```python
from build123d import *

# Parameters (mm, degrees)
BOSS_EXTRUDE1_DEPTH             = 7.62
SKETCH1_3_R                     = 1.5
BOSS_EXTRUDE2_DEPTH             = 2.54
SKETCH2_W                       = 63.119
SKETCH2_H                       = 7.62
BOSS_EXTRUDE3_DEPTH             = 2.54
BOSS_EXTRUDE3_DIRECTION_2_REACH = 58.274
FILLET1_R                       = 15.24
FILLET2_R                       = 5.08
FILLET3_R                       = 2.54


with BuildPart() as part:
    # Sketch1 → Boss-Extrude1 (new body)
    with BuildSketch(Plane.XY):
        with BuildLine():
            Line((-37.554226409, 19.773329444), (-37.554226409, 16.344329444))
            Line((-37.554226409, 16.344329444), (-8.344226409, 16.344329444))
            ThreePointArc((-8.344226409, 16.344329444), (-0.261995901, 12.996559953), (3.085773591, 4.914329444))
            Line((3.085773591, 4.914329444), (3.085773591, -14.770670556))
            Line((3.085773591, -14.770670556), (-37.554226409, -14.770670556))
            Line((-37.554226409, -14.770670556), (-37.554226409, -21.438170556))
            Line((-37.554226409, -21.438170556), (6.514773591, -21.438170556))
            Line((6.514773591, -21.438170556), (25.564773591, -21.120670556))
            Line((25.564773591, -21.120670556), (6.514773591, -6.642670556))
            Line((6.514773591, -6.642670556), (6.514773591, 4.914329444))
            ThreePointArc((6.514773591, 4.914329444), (2.162673252, 15.421229106), (-8.344226409, 19.773329444))
            Line((-8.344226409, 19.773329444), (-37.554226409, 19.773329444))
        make_face()
    extrude(amount=-BOSS_EXTRUDE1_DEPTH)

    # Sketch1<3> → Boss-Extrude2 (add)
    with BuildSketch(Plane.XY):
        with BuildLine():
            Line((-8.344226409, 16.344329444), (-37.554226409, 16.344329444))
            Line((-37.554226409, 16.344329444), (-37.554226409, -14.770670556))
            Line((-37.554226409, -14.770670556), (3.085773591, -14.770670556))
            Line((3.085773591, -14.770670556), (3.085773591, 4.914329444))
            ThreePointArc((3.085773591, 4.914329444), (-0.261995901, 12.996559953), (-8.344226409, 16.344329444))
        make_face()
        with Locations((-29.732882342, -7.215397763)):
            Circle(SKETCH1_3_R, mode=Mode.SUBTRACT)
        with Locations((-4.332882342, -7.215397763)):
            Circle(SKETCH1_3_R, mode=Mode.SUBTRACT)
        with Locations((-29.710505244, 10.645398587)):
            Circle(SKETCH1_3_R, mode=Mode.SUBTRACT)
        with Locations((-4.310505244, 10.645398587)):
            Circle(SKETCH1_3_R, mode=Mode.SUBTRACT)
    extrude(amount=-BOSS_EXTRUDE2_DEPTH)

    # Sketch2 → Boss-Extrude3 (add)
    with BuildSketch(Plane.XZ.offset(21.438170556)):
        with Locations((-5.994726409, -3.81)):
            Rectangle(SKETCH2_W, SKETCH2_H)
    extrude(amount=BOSS_EXTRUDE3_DEPTH)

    # Boss-Extrude3 direction 2: up to this face of the body (flat: up to its plane)
    boss_extrude3_direction_2_end = Plane(part.part.faces().sort_by_distance((16.039773591, -21.279420556, -3.81))[0])
    # Sketch2 → Boss-Extrude3 direction 2 (add, up to the picked face)
    with BuildSketch(Plane.XZ.offset(21.438170556), mode=Mode.PRIVATE) as boss_extrude3_direction_2_sk1:
        with Locations((-5.994726409, -3.81)):
            Rectangle(SKETCH2_W, SKETCH2_H)
    boss_extrude3_direction_2_tool1 = split(extrude(boss_extrude3_direction_2_sk1.sketch, amount=-BOSS_EXTRUDE3_DIRECTION_2_REACH, mode=Mode.PRIVATE), bisect_by=boss_extrude3_direction_2_end, keep=Keep.BOTH, mode=Mode.PRIVATE)
    add(boss_extrude3_direction_2_tool1.solids().sort_by(Axis((-5.994726, -21.438171, -3.81), (0, 1, 0)))[0])

    # Fillet1
    fillet1_edges = [part.edges().sort_by_distance(p)[0] for p in [
        (-37.554226409, 19.773329444, -3.81),
        (-37.554226409, -23.978170556, -3.81),
    ]]
    fillet(fillet1_edges, radius=FILLET1_R)

    # Fillet2
    fillet2_edges = [part.edges().sort_by_distance(p)[0] for p in [
        (25.564773591, -21.120670556, -3.81),
    ]]
    fillet(fillet2_edges, radius=FILLET2_R)

    # Fillet3
    fillet3_edges = [part.edges().sort_by_distance(p)[0] for p in [
        (6.514773591, -6.642670556, -3.81),
    ]]
    fillet(fillet3_edges, radius=FILLET3_R)


solid = part.part
```
The model under review builds one solid part; all positions refer to its coordinate system, in mm. A direction names the side the tool comes from. Give positions to 0.01 mm unless a question says otherwise; leave off trailing zeros. Write each loop counter-clockwise with the first axis right and the second up, starting at its lowest first coordinate (ties: lowest second). Pieces come first, ordered by that corner, then holes.
(1) The part is to be moulded in two halves that separate along Y. For faces 1 (the flat face through (3.086, -5, -5)), 2 (the cylindrical face through (6.79, -6.53, -3.86)), 3 (the flat face through (-6, -15, -7.62)), say which applies: released by +Y, released by -Y, zero draft, split by the parting line, or undercut.
(2) Consider section D-D, the plane y = -3.5. Give the boundary of the cut face in (x, z), and give its area (3 significant figures).
(3) To check wall thickness, follow L1, parallel to Y at x = -13, z = -3; L2, parallel to Z at x = -12.5, y = -8.5; L3, parallel to Y at x = 0.5, z = -4. State the ranges of each line that lie inside material, in increasing order.
(4) Tool access review of faces 4 (the flat face through (-20, 16.344, -5)), 5 (the cylindrical face through (-28.302, -6.765, -1.252)): name each direction out of +Z, -Z, +X, -X, +Y, -Y from which nothing blocks a thin tool from reaching the whole face with its end or side.
(5) For P1, Ø25, axis at x = -9.5, y = 6.5, coming from the -Z side; P2, Ø3.5, axis at x = -4.31, y = 10.65, coming from the -Z side; P3, Ø4, axis at y = -10, z = -5.5, coming from the -X side; P4, Ø4, axis at y = 1.5, z = -5.5, coming from the +X side, all flat-tipped, find the tip position at first contact; note any pin that passes through.
(6) Consider section A-A, the plane x = -4.5. Give the boundary of the cut face in (y, z), and give its area (3 significant figures).
(7) Consider section C-C, the plane y = 8.5. Give the boundary of the cut face in (x, z).
(8) Consider section B-B, the plane z = -3.5. Give the boundary of the cut face in (x, y).
Returned:
1. face 1: undercut
1. face 2: released by +Y
1. face 3: zero draft
2. outline: (-37.55, -2.54) - (3.09, -2.54) - (3.09, -7.62) - (6.51, -7.62) - (6.51, 0) - (-37.55, 0) - close
2. area: 129 mm2
3. L1: y = -23.98 to -14.77, 16.34 to 19.77
3. L2: z = -2.54 to 0
3. L3: y = -23.98 to -14.77, 12.15 to 16.85
4. face 4: -Z, -X
4. face 5: +Z, -Z
5. P1: stops at z = -7.62
5. P2: stops at z = -2.54
5. P3: stops at x = 3.09
5. P4: stops at x = 6.51
6. outline: (-23.98, -7.62) - (-14.77, -7.62) - (-14.77, -2.54) - (-8.71, -2.54) - (-8.71, 0) - (-23.98, 0) - close; (-5.72, -2.54) - (9.16, -2.54) - (9.16, 0) - (-5.72, 0) - close; (12.13, -2.54) - (15.68, -2.54) - (15.68, -7.62) - (19.27, -7.62) - (19.27, 0) - (12.13, 0) - close
6. area: 160 mm2
7. outline: (-37.03, -2.54) - (2.51, -2.54) - (2.51, -7.62) - (6.08, -7.62) - (6.08, 0) - (-37.03, 0) - close
8. outline: (-36.31, -14.77) arc R15.24 ccw to (-22.31, -23.98) - (25.56, -23.98) - (25.56, -23.64) arc R5.08 ccw to (23.56, -19.6) - (7.52, -7.41) arc R2.54 cw to (6.51, -5.38) - (6.51, 4.91) arc R14.86 ccw to (-8.34, 19.77) - (-22.31, 19.77) arc R15.24 ccw to (-31.95, 16.34) - (-8.34, 16.34) arc R11.43 cw to (3.09, 4.91) - (3.09, -14.77) - close
